For this review, take the finished solid that the model builds, in its own axes (mm). Face numbers are marked on the shaded views. Give positions to 0.01 mm unless a question says otherwise; leave off trailing zeros. Order: outer loops, then holes, each group sorted by start corner. A loop starts at its lowest first (then second) coordinate and runs counter-clockwise, first axis right, second up. Notation, with made-up numbers: (-22.75, 51.25) - (11.25, 51.25) arc R34 cw to (11.25, 86.25) - close; hole circle Ø2 at (27, -26.75). An arc over 180 degrees is marked (long way). Use a Markdown table: item, result. Add a question column.
1) We need section D-D on x = 657. Write out the cut boundary in (y, z), then the cut area to 3 significant figures.
2) Wall thickness on L1, parallel to Y at x = 658.5, z = 1268.75; L2, parallel to Y at x = 679, z = 1266; L3, parallel to X at y = 887, z = 1265.5: over which ranges is each line inside the solid? List them lowest first.
3) We need section A-A on x = 693. Write out the cut boundary in (y, z), then the cut area to 3 significant figures.
4) Mouldability with a two-part tool opening along X and no side actions: class the marked faces 1 and 2 as released by +X, released by -X, zero draft, split by the parting line, or undercut.
5) Clearance check with flat-ended pins moving along their axes: P1, Ø6, axis at x = 664, z = 1262, coming from the +Y side; P2, Ø2, axis at x = 672.5, z = 1266, coming from the -Y side; P3, Ø6, axis at x = 716.94, y = 897.34, coming from the -Z side; P4, Ø2.5, axis at x = 620.34, y = 912.34, coming from the +Z side. State where each tip first meets the part, or that it passes through.
6) We need section C-C on z = 1255. Write out the cut boundary in (x, y).
7) We need section B-B on y = 875.5. Write out the cut boundary in (x, z).
```python
from build123d import *

# Parameters (mm, degrees)
BOSS_EXTRUDE1_DEPTH           = 1
BOSS_EXTRUDE2_START           = 4
BOSS_EXTRUDE2_DEPTH           = 4
BOSS_EXTRUDE3_START           = 1
BOSS_EXTRUDE3_DEPTH           = 1
CBORE_FOR_M3_SHCS1_AT_2_COUNT = 2
CBORE_FOR_M3_SHCS1_AT_2_PITCH = 143.8
CBORE_FOR_M3_SHCS1_AT_3_COUNT = 2
CBORE_FOR_M3_SHCS1_AT_3_PITCH = 150.091438796
CBORE_FOR_M3_SHCS1_AT_4_COUNT = 2
CBORE_FOR_M3_SHCS1_AT_4_PITCH = 43
BOSS_EXTRUDE4_START           = -6
BOSS_EXTRUDE4_OUTLINE_R       = 1.7
BOSS_EXTRUDE4_DEPTH           = 6
BOSS_EXTRUDE5_DEPTH           = 20


# Read off the part's stored shape, not the designer's step: Boss-Extrude4
with BuildPart() as part:
    # Sketch1 → Boss-Extrude1 (new body)
    with BuildSketch(Plane(origin=(0, 0, 1268.319699828), x_dir=(-1, 0, 0), z_dir=(0, 0, -1))):
        with BuildLine():
            Line((-565.344205178, 854.342421724), (-565.344205178, 897.342374326))
            ThreePointArc((-565.344205178, 897.342374326), (-567.628754858, 902.85784955), (-573.144231788, 905.142395114))
            Line((-573.144231788, 905.142395114), (-716.944184389, 905.142395114))
            ThreePointArc((-716.944184389, 905.142395114), (-722.459659614, 902.857845434), (-724.744205178, 897.342368505))
            Line((-724.744205178, 897.342368505), (-724.744205178, 854.342415903))
            ThreePointArc((-724.744205178, 854.342415903), (-722.459655498, 848.826940679), (-716.944178568, 846.542395115))
            Line((-716.944178568, 846.542395115), (-573.144231788, 846.542395115))
            ThreePointArc((-573.144231788, 846.542395115), (-567.6287528, 848.826942737), (-565.344205178, 854.342421724))
        make_face()
        with BuildLine():
            Line((-568.344205178, 854.342399549), (-568.344205178, 897.342395114))
            ThreePointArc((-568.344205178, 897.342395114), (-569.750074712, 900.736528717), (-573.144209613, 902.142395114))
            Line((-573.144209613, 902.142395114), (-716.944205178, 902.142395114))
            ThreePointArc((-716.944205178, 902.142395114), (-720.33833878, 900.736525581), (-721.744205178, 897.342390679))
            Line((-721.744205178, 897.342390679), (-721.744205178, 854.342395114))
            ThreePointArc((-721.744205178, 854.342395114), (-720.338335644, 850.948261512), (-716.944200743, 849.542395115))
            Line((-716.944200743, 849.542395115), (-573.144209613, 849.542395115))
            ThreePointArc((-573.144209613, 849.542395115), (-569.750073144, 850.94826308), (-568.344205178, 854.342399549))
        make_face(mode=Mode.SUBTRACT)
    extrude(amount=-BOSS_EXTRUDE1_DEPTH)

    # Sketch2 → Boss-Extrude2 (add)
    with BuildSketch(Plane(origin=(0, 0, 1268.319699828), x_dir=(-1, 0, 0), z_dir=(0, 0, -1)).offset(BOSS_EXTRUDE2_START)):
        with BuildLine():
            Line((-565.344205178, 854.342421724), (-565.344205178, 897.342374326))
            ThreePointArc((-565.344205178, 897.342374326), (-567.628754858, 902.85784955), (-573.144231788, 905.142395114))
            Line((-573.144231788, 905.142395114), (-716.944184389, 905.142395114))
            ThreePointArc((-716.944184389, 905.142395114), (-722.459659614, 902.857845434), (-724.744205178, 897.342368505))
            Line((-724.744205178, 897.342368505), (-724.744205178, 854.342415903))
            ThreePointArc((-724.744205178, 854.342415903), (-722.459655498, 848.826940679), (-716.944178568, 846.542395115))
            Line((-716.944178568, 846.542395115), (-573.144231788, 846.542395115))
            ThreePointArc((-573.144231788, 846.542395115), (-567.6287528, 848.826942737), (-565.344205178, 854.342421724))
        make_face()
        with BuildLine():
            Line((-573.344205178, 864.542395115), (-573.344205178, 887.142395114))
            ThreePointArc((-573.344205178, 887.142395114), (-576.273137366, 894.213462926), (-583.344205178, 897.142395114))
            Line((-583.344205178, 897.142395114), (-706.744205178, 897.142395114))
            ThreePointArc((-706.744205178, 897.142395114), (-713.81527299, 894.213462926), (-716.744205178, 887.142395114))
            Line((-716.744205178, 887.142395114), (-716.744205178, 864.542395115))
            ThreePointArc((-716.744205178, 864.542395115), (-713.81527299, 857.471327303), (-706.744205178, 854.542395115))
            Line((-706.744205178, 854.542395115), (-583.344205178, 854.542395115))
            ThreePointArc((-583.344205178, 854.542395115), (-576.273137366, 857.471327303), (-573.344205178, 864.542395115))
        make_face(mode=Mode.SUBTRACT)
    extrude(amount=-BOSS_EXTRUDE2_DEPTH)

    # Sketch3 → Boss-Extrude3 (add)
    with BuildSketch(Plane(origin=(0, 0, 1264.319699828), x_dir=(-1, 0, 0), z_dir=(0, 0, -1)).offset(BOSS_EXTRUDE3_START)):
        with BuildLine():
            Line((-565.344205178, 854.342421724), (-565.344205178, 897.342374326))
            ThreePointArc((-565.344205178, 897.342374326), (-567.628754858, 902.85784955), (-573.144231788, 905.142395114))
            Line((-573.144231788, 905.142395114), (-716.944184389, 905.142395114))
            ThreePointArc((-716.944184389, 905.142395114), (-722.459659614, 902.857845434), (-724.744205178, 897.342368505))
            Line((-724.744205178, 897.342368505), (-724.744205178, 854.342415903))
            ThreePointArc((-724.744205178, 854.342415903), (-722.459655498, 848.826940679), (-716.944178568, 846.542395115))
            Line((-716.944178568, 846.542395115), (-573.144231788, 846.542395115))
            ThreePointArc((-573.144231788, 846.542395115), (-567.6287528, 848.826942737), (-565.344205178, 854.342421724))
        make_face()
    extrude(amount=-BOSS_EXTRUDE3_DEPTH)

    # Sketch5 → CBORE for M3 SHCS1 (revolve, cut)
    with BuildSketch(Plane(origin=(716.944205178, 897.342395114, 1263.319699828), x_dir=(0, 1, 0), z_dir=(1, 0, 0))):
        Polygon((0, 0), (0, 6), (1.7, 6), (1.7, 3), (3.25, 3), (3.25, 0.025), (3.275, 0), align=None)
    cbore_for_m3_shcs1 = revolve(axis=Axis((716.944205178, 897.342395114, 1256.969699828), (0, 0, 1)), mode=Mode.SUBTRACT)

    # CBORE for M3 SHCS1 at 2: CBORE for M3 SHCS1 ×2
    with Locations(*[(-i * CBORE_FOR_M3_SHCS1_AT_2_PITCH, 0, 0) for i in range(1, CBORE_FOR_M3_SHCS1_AT_2_COUNT)]):
        add(cbore_for_m3_shcs1, mode=Mode.SUBTRACT)

    # CBORE for M3 SHCS1 at 3: CBORE for M3 SHCS1 ×2
    with Locations(*[Vector(-0.958082627184226, -0.2864920234278285, 0) * (i * CBORE_FOR_M3_SHCS1_AT_3_PITCH) for i in range(1, CBORE_FOR_M3_SHCS1_AT_3_COUNT)]):
        add(cbore_for_m3_shcs1, mode=Mode.SUBTRACT)

    # CBORE for M3 SHCS1 at 4: CBORE for M3 SHCS1 ×2
    with Locations(*[(0, -i * CBORE_FOR_M3_SHCS1_AT_4_PITCH, 0) for i in range(1, CBORE_FOR_M3_SHCS1_AT_4_COUNT)]):
        add(cbore_for_m3_shcs1, mode=Mode.SUBTRACT)


with BuildPart() as boss_extrude4_tool:
    # Boss-Extrude4 outline → Boss-Extrude4 (new body)
    # profile 1 of 2: a face of its own
    with BuildSketch(Plane(origin=(0, 0, 1263.319699828), x_dir=(-1, 0, 0), z_dir=(0, 0, -1)).offset(BOSS_EXTRUDE4_START)):
        with BuildLine():
            ThreePointArc((-635.044202268, 846.542389294), (-629.953035501, 844.433558971), (-627.844205178, 839.342392204))
            ThreePointArc((-627.844205178, 839.342392204), (-620.344205178, 831.842392204), (-612.844205178, 839.342392204))
            ThreePointArc((-612.844205178, 839.342392204), (-610.735374855, 844.433558971), (-605.644208088, 846.542389294))
            Line((-605.644208088, 846.542389294), (-635.044202268, 846.542389294))
        make_face()
        with Locations((-620.344205178, 839.342392204)):
            Circle(BOSS_EXTRUDE4_OUTLINE_R, mode=Mode.SUBTRACT)
    # profile 2 of 2: a face of its own
    with BuildSketch(Plane(origin=(0, 0, 1263.319699828), x_dir=(-1, 0, 0), z_dir=(0, 0, -1)).offset(BOSS_EXTRUDE4_START)):
        with BuildLine():
            ThreePointArc((-605.644208088, 905.142395114), (-610.735374855, 907.251225437), (-612.844205178, 912.342392204))
            ThreePointArc((-612.844205178, 912.342392204), (-620.344205178, 919.842392204), (-627.844205178, 912.342392204))
            ThreePointArc((-627.844205178, 912.342392204), (-629.953035501, 907.251225437), (-635.044202268, 905.142395114))
            Line((-635.044202268, 905.142395114), (-605.644208088, 905.142395114))
        make_face()
        with Locations((-620.344205178, 912.342392204)):
            Circle(BOSS_EXTRUDE4_OUTLINE_R, mode=Mode.SUBTRACT)
    extrude(amount=BOSS_EXTRUDE4_DEPTH)


with BuildPart() as part_1:
    add(part.part)


with BuildPart() as part_2:
    # Boss-Extrude4: joined with boss_extrude4_tool
    add(part_1.part.fuse(boss_extrude4_tool.part, tol=0.00001))

    # Sketch7 → Boss-Extrude5 (add)
    with BuildSketch(Plane(origin=(655.044202268, 0, 0), x_dir=(0, 0, -1), z_dir=(1, 0, 0))):
        with BuildLine():
            Line((-1263.319699828, 849.042392204), (-1256.519699828, 849.042392204))
            Line((-1256.519699828, 849.042392204), (-1256.519699828, 846.042392204))
            Line((-1256.519699828, 846.042392204), (-1253.519699828, 846.042392204))
            Line((-1253.519699828, 846.042392204), (-1253.519699828, 854.042392204))
            Line((-1253.519699828, 854.042392204), (-1258.319699828, 854.042392204))
            ThreePointArc((-1258.319699828, 854.042392204), (-1261.855233734, 855.506858298), (-1263.319699828, 859.042392204))
            Line((-1263.319699828, 859.042392204), (-1263.319699828, 849.042392204))
        make_face()
    extrude(amount=BOSS_EXTRUDE5_DEPTH)


solid = part_2.part
```
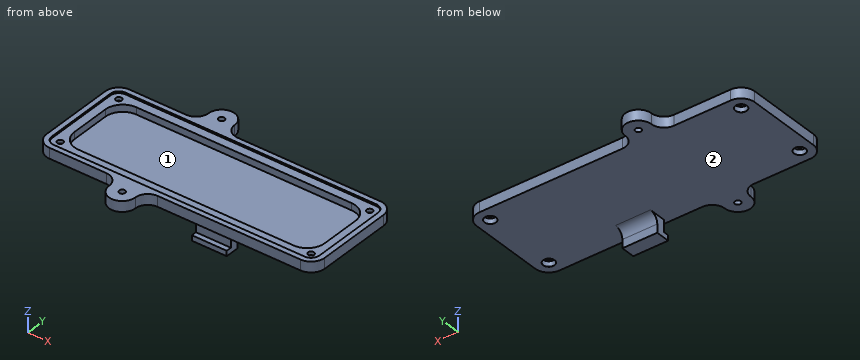
Checked values:
| question | item | result |
|---|---|---|
| 1 | outline | (846.04, 1253.52) - (854.04, 1253.52) - (854.04, 1258.32) arc R5 cw to (859.04, 1263.32) - (905.14, 1263.32) - (905.14, 1269.32) - (902.14, 1269.32) - (902.14, 1268.32) - (897.14, 1268.32) - (897.14, 1264.32) - (854.54, 1264.32) - (854.54, 1268.32) - (849.54, 1268.32) - (849.54, 1269.32) - (846.54, 1269.32) - (846.54, 1263.32) - (849.04, 1263.32) - (849.04, 1256.52) - (846.04, 1256.52) - close |
| 1 | area | 192 mm² |
| 2 | L1 | 846.54 to 849.54, 902.14 to 905.14 |
| 2 | L2 | 846.54 to 854.54, 897.14 to 905.14 |
| 2 | L3 | 565.34 to 573.34, 716.74 to 724.74 |
| 3 | outline | (846.54, 1263.32) - (905.14, 1263.32) - (905.14, 1269.32) - (902.14, 1269.32) - (902.14, 1268.32) - (897.14, 1268.32) - (897.14, 1264.32) - (854.54, 1264.32) - (854.54, 1268.32) - (849.54, 1268.32) - (849.54, 1269.32) - (846.54, 1269.32) - close |
| 3 | area | 129 mm² |
| 4 | face 1 | undercut |
| 4 | face 2 | zero draft |
| 5 | P1 | y = 905.14 |
| 5 | P2 | y = 846.54 |
| 5 | P3 | z = 1266.32 |
| 5 | P4 | through |
| 6 | outline | (655.04, 846.04) - (675.04, 846.04) - (675.04, 854.04) - (655.04, 854.04) - close |
| 7 | outline | (565.34, 1263.32) - (724.74, 1263.32) - (724.74, 1269.32) - (721.74, 1269.32) - (721.74, 1268.32) - (716.74, 1268.32) - (716.74, 1264.32) - (573.34, 1264.32) - (573.34, 1268.32) - (568.34, 1268.32) - (568.34, 1269.32) - (565.34, 1269.32) - close |
